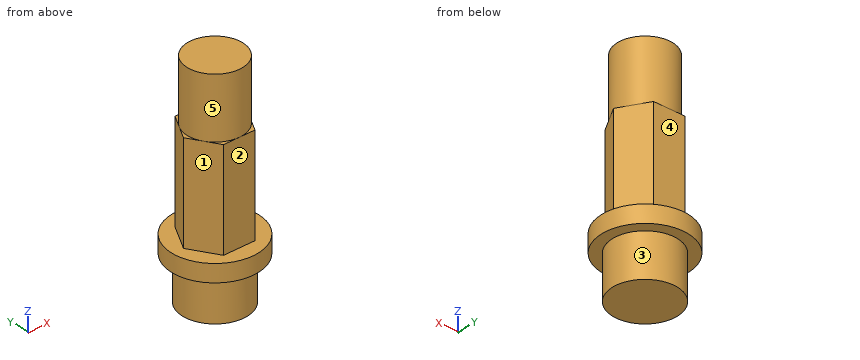
from build123d import *

# Parameters (mm, degrees)
SKETCH1_R           = 3.75
BOSS_EXTRUDE1_DEPTH = 5
SKETCH2_R           = 5
BOSS_EXTRUDE2_DEPTH = 2
BOSS_EXTRUDE3_DEPTH = 11.4
SKETCH4_R           = 3.204293994
BOSS_EXTRUDE4_DEPTH = 7


with BuildPart() as part:
    # Sketch1 → Boss-Extrude1 (new body)
    with BuildSketch(Plane.XY):
        Circle(SKETCH1_R)
    extrude(amount=BOSS_EXTRUDE1_DEPTH)

    # Sketch2 → Boss-Extrude2 (add)
    with BuildSketch(Plane.XY.offset(5)):
        Circle(SKETCH2_R)
    extrude(amount=BOSS_EXTRUDE2_DEPTH)

    # Sketch3 → Boss-Extrude3 (add)
    with BuildSketch(Plane.XY.offset(7)):
        Polygon((3.7, 0), (1.85, 3.204293994), (-1.85, 3.204293994), (-3.7, 0), (-1.85, -3.204293994), (1.85, -3.204293994), align=None)
    extrude(amount=BOSS_EXTRUDE3_DEPTH)

    # Sketch4 → Boss-Extrude4 (add)
    with BuildSketch(Plane.XY.offset(18.4)):
        Circle(SKETCH4_R)
    extrude(amount=BOSS_EXTRUDE4_DEPTH)


solid = part.part
Check sheet for the modelled part. Datum: model origin and axes. Units: mm. Face numbers are marked on the shaded views. A direction names the side the tool comes from. Round coordinates to 2 decimals unless told otherwise and drop trailing zeros. Write each loop counter-clockwise with the first axis right and the second up, starting at its lowest first coordinate (ties: lowest second). Pieces come first, ordered by that corner, then holes. Notation, with made-up numbers: (-28, -19.5) -> (16, -19.5) arc R25 ccw to (16, 16.5) -> close; hole circle Ø11 at (-28, 32). An arc over 180 degrees is marked (long way). Answer as CSV lines item,"result". Start each with the question number.
1) Material ranges on line 1 (Y direction, x = -0.5, z = 14.75); line 2 (Z direction, x = -4.5, y = -1.75); line 3 (X direction, y = 2, z = 20), recorded low to high. Write a range as from..to.
2) Tool access check on the marked faces 1, 2, 3, 4 and 5. Record the directions out of +Z, -Z, +X, -X, +Y, -Y that give a thin tool (end or side, any length) a straight path to the whole face; none if there is none.
3) Section check D-D on z = 5.5. Enter the section's corners in (x, y).
4) Section check C-C on y = -2. Enter the section's corners in (x, z), and give its area (3 significant figures).
5) Section check A-A on z = 9. Enter the section's corners in (x, y), and give its area (3 significant figures).
6) Section check B-B on x = 1.5. Enter the section's corners in (y, z).
7) Go/stop test with flat-tipped pins: P1, Ø1.8, axis at x = 0, z = 15, coming from the +Y side; P2, Ø2, axis at x = -4, y = 3, coming from the -Z side; P3, Ø4, axis at x = 1, z = 13, coming from the -Y side. Record where each tip stops, or that it passes through.
Found:
1,line 1,"y = -3.2..3.2"
1,line 2,"z = 5..7"
1,line 3,"x = -2.5..2.5"
2,face 1,"+Z, -X, -Y"
2,face 2,"+Z, +X, -X, -Y"
2,face 3,"-Z"
2,face 4,"+Z, +X, -X, +Y"
2,face 5,"+Z"
3,outline,"circle Ø10 at (0, 0)"
4,outline,"(-4.58, 5) -> (-3.17, 5) -> (-3.17, 0) -> (3.17, 0) -> (3.17, 5) -> (4.58, 5) -> (4.58, 7) -> (2.55, 7) -> (2.55, 18.4) -> (2.5, 18.4) -> (2.5, 25.4) -> (-2.5, 25.4) -> (-2.5, 18.4) -> (-2.55, 18.4) -> (-2.55, 7) -> (-4.58, 7) -> close"
4,area,"143 mm^2"
5,outline,"(-3.7, 0) -> (-1.85, -3.2) -> (1.85, -3.2) -> (3.7, 0) -> (1.85, 3.2) -> (-1.85, 3.2) -> close"
5,area,"35.6 mm^2"
6,outline,"(-4.77, 5) -> (-3.44, 5) -> (-3.44, 0) -> (3.44, 0) -> (3.44, 5) -> (4.77, 5) -> (4.77, 7) -> (3.2, 7) -> (3.2, 18.4) -> (2.83, 18.4) -> (2.83, 25.4) -> (-2.83, 25.4) -> (-2.83, 18.4) -> (-3.2, 18.4) -> (-3.2, 7) -> (-4.77, 7) -> close"
7,P1,"stops at y = 3.2"
7,P2,"stops at z = 5"
7,P3,"stops at y = -3.2"
